```python
from build123d import *

# Parameters (mm, degrees)
F2_R      = 20
F3_DEPTH  = 61.6
F5_R      = 30
F5_R_2    = 20
F6_DEPTH  = 35
F7_R      = 27.5
F7_R_2    = 20
F8_DEPTH  = 20
F9_R      = 25
F10_W     = 8
F10_H     = 13.5
F11_DEPTH = 17.5
F12_W     = 8
F12_H     = 13.5


with BuildPart() as f1:
    # F0 (on Front) → F1 (revolve)
    with BuildSketch(Plane.XZ):
        with BuildLine():
            ThreePointArc((40, 0), (0, 40), (-40, 0))
            Line((-40, 0), (40, 0))
        make_face()
    revolve(axis=Axis((0, 0, 0), (1, 0, 0)))

    # F2 (on Right) → F3 (cut)
    with BuildSketch(Plane.YZ):
        Circle(F2_R)
    extrude(amount=F3_DEPTH, mode=Mode.SUBTRACT)

    # F5 (on Right) → F6 (join)
    with BuildSketch(Plane.YZ):
        Circle(F5_R)
        Circle(F5_R_2, mode=Mode.SUBTRACT)
    extrude(amount=F6_DEPTH)

    # F7 (on face) → F8 (cut)
    with BuildSketch(Plane.YZ.offset(35)):
        Circle(F7_R)
        Circle(F7_R_2, mode=Mode.SUBTRACT)
    extrude(amount=-F8_DEPTH, mode=Mode.SUBTRACT)

    # F9
    f9_edges = [f1.edges().sort_by_distance(p)[0] for p in [
        (26.457513, 21.213203, 21.213203),
        (26.457513, -21.213203, -21.213203),
    ]]
    fillet(f9_edges, radius=F9_R)

    # F10 (on face) → F11 (cut)
    with BuildSketch(Plane.YZ):
        with BuildLine():
            ThreePointArc((3.8518622015, 13.5), (-0.1481377985, 17.5), (-4.1481377985, 13.5))
            Line((-4.1481377985, 13.5), (3.8518622015, 13.5))
        make_face()
        with Locations((-0.1481377985, 6.75)):
            Rectangle(F10_W, F10_H)
        with Locations((-0.1481377985, -6.75)):
            Rectangle(F10_W, F10_H)
        with BuildLine():
            Line((3.8518622015, -13.5), (-4.1481377985, -13.5))
            ThreePointArc((-4.1481377985, -13.5), (-0.1481377985, -17.5), (3.8518622015, -13.5))
        make_face()
    extrude(amount=-F11_DEPTH, mode=Mode.SUBTRACT)

    # F12 (on face) → F13 (revolve, cut)
    with BuildSketch(Plane.YZ.offset(-17.5)):
        with BuildLine():
            ThreePointArc((3.8518622015, 13.5), (-0.1481377985, 17.5), (-4.1481377985, 13.5))
            Line((-4.1481377985, 13.5), (3.8518622015, 13.5))
        make_face()
        with Locations((-0.1481377985, 6.75)):
            Rectangle(F12_W, F12_H)
    revolve(axis=Axis((-17.5, -0.1481377985, 0), (0, -1, 0)), mode=Mode.SUBTRACT)


solid = f1.part
```
Design review of the part built by this model. Coordinates are the model's own, in mm. Round coordinates to 2 decimals unless told otherwise and drop trailing zeros. Write each loop counter-clockwise with the first axis right and the second up, starting at its lowest first coordinate (ties: lowest second). Pieces come first, ordered by that corner, then holes. Notation, with made-up numbers: (5, 82.25) -> (16, 82.25) arc R27 ccw to (16, 102.25) -> close; hole circle Ø9 at (60.25, 5). An arc over 180 degrees is marked (long way). Answer in a Markdown table with one row per item.
Q1. Draft analysis for pull direction Z (two halves, no side actions). For faces 1 (the face through (34.814, 28.615, 9.011)), 2 (the face through (15, 1.9, -20.2)), 3 (the face through (35, 13.2, -24.3)), state which applies: +Z half, -Z half, draft (parallel to the pull), parting line (faces both ways), or undercut.
The answers:
| item | result |
|---|---|
| face 1 | parting line |
| face 2 | undercut |
| face 3 | draft |
Q2. Clearance check with flat-ended pins moving along their axes: pin 1 Ø5 at (y, z) = (21, 28) entering from -X; pin 2 Ø2 at (x, y) = (18.5, -7.5) entering from +Z; pin 3 Ø2 at (x, z) = (-20.5, 28) entering from +Y. State where each tip first meets the part, or that it passes through.
The answers:
| item | result |
|---|---|
| pin 1 | x = -23.32 |
| pin 2 | z = 35.22 |
| pin 3 | y = 21.54 |
Q3. To check wall thickness, follow L1, parallel to Y at x = 22, z = -6; L2, parallel to Z at x = 26.5, y = -5; L3, parallel to Y at x = 18, z = 9.5. State the ranges of each line that lie inside material, in increasing order. Write a range as [from, to].
The answers:
| item | result |
|---|---|
| L1 | [-32.89, -26.84], [26.84, 32.89] |
| L2 | [-30.96, -27.04], [27.04, 30.96] |
| L3 | [-34.43, -25.81], [25.81, 34.43] |
Q4. Take a section at B-B, the plane x = 12.5. State the section outline as (y, z) points, then the cut area to 3 significant figures.
The answers:
| item | result |
|---|---|
| outline | circle Ø75.99 at (0, 0); hole circle Ø40 at (0, 0) |
| area | 3,280 mm² |
Q5. Take a section at A-A, the plane x = -2. State the section outline as (y, z) points, then the cut area to 3 significant figures.
The answers:
| item | result |
|---|---|
| outline | circle Ø79.9 at (0, 0); hole (-4.15, -13.5) arc R4 ccw to (3.85, -13.5) -> (3.85, 13.5) arc R4 ccw to (-4.15, 13.5) -> close |
| area | 4,750 mm² |
